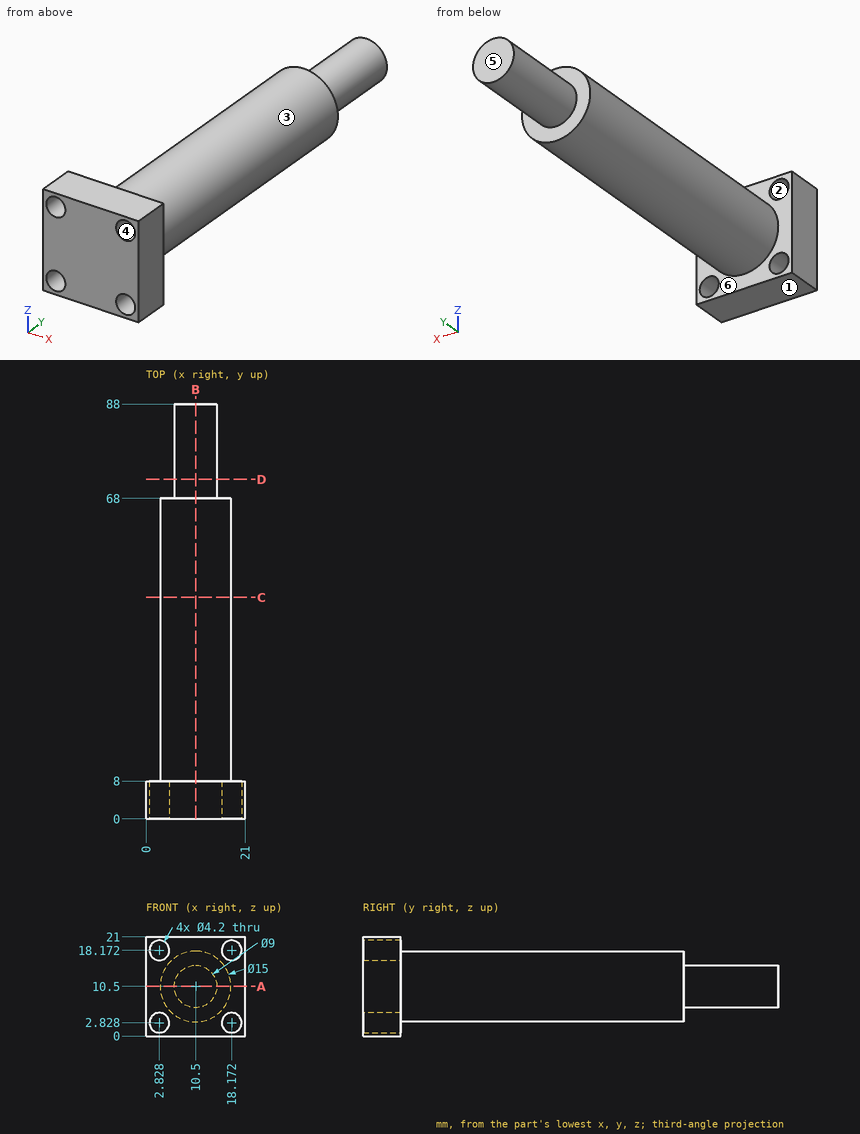
Verification items for this drawing (mm, ordinates from the low corner). A direction names the side the tool comes from. Coordinates: 2 decimals unless noted, no trailing zeros. Order: outer loops, then holes, each group sorted by start corner. A loop starts at its lowest first (then second) coordinate and runs counter-clockwise, first axis right, second up.
Q1. Sectioned sample at D-D on y = 72. Record the cut outline in (x, z).
Reply:
outline: circle Ø9 at (10.5, 10.5)
Q2. Sectioned sample at C-C on y = 47. Record the cut outline in (x, z).
Reply:
outline: circle Ø15 at (10.5, 10.5)
Q3. Depth check by flat-ended pin: pin 1 Ø10 at (x, y) = (18, 59.5) entering from -Z; pin 2 Ø2 at (x, y) = (10, 43.5) entering from +Z; pin 3 Ø3 at (x, z) = (4, 4.5) entering from +Y. Enter the tip coordinate at first touch or a pass-through.
Reply:
pin 1: stops at z = 3.43
pin 2: stops at z = 18
pin 3: stops at y = 68
Q4. Tool access check on the marked faces 5 and 6. Record the directions out of +Z, -Z, +X, -X, +Y, -Y that give a thin tool (end or side, any length) a straight path to the whole face; none if there is none.
Reply:
face 5: +Z, -Z, +X, -X, +Y
face 6: +Y
Q5. Thickness scan on probe 1 along Z at (x, y) = (11, 31); probe 2 along Y at (x, z) = (14, 5); probe 3 along Y at (x, z) = (3.75, 15.75). Record the ranges inside material, lowest first.
Reply:
probe 1: z = 3.02 to 17.98
probe 2: y = 0 to 68
probe 3: y = 0 to 8
Q6. Draft check along Z on the marked faces 1, 2, 3 and 4. Enter one of: released by +Z, released by -Z, zero draft, split by the parting line, or undercut.
Reply:
face 1: released by -Z
face 2: undercut
face 3: split by the parting line
face 4: undercut
Q7. Sectioned sample at B-B on x = 10.5. Record the cut outline in (y, z), and give its area (3 significant figures).
Reply:
outline: (0, 0) - (8, 0) - (8, 3) - (68, 3) - (68, 6) - (88, 6) - (88, 15) - (68, 15) - (68, 18) - (8, 18) - (8, 21) - (0, 21) - close
area: 1,250 mm2
Q8. Sectioned sample at A-A on z = 10.5. Record the cut outline in (x, y), and give its area (3 significant figures).
Reply:
outline: (0, 0) - (21, 0) - (21, 8) - (18, 8) - (18, 68) - (15, 68) - (15, 88) - (6, 88) - (6, 68) - (3, 68) - (3, 8) - (0, 8) - close
area: 1,250 mm2
